from build123d import *

# Parameters (mm, degrees)
BOSS_EXTRUDE1_DEPTH     = 4
SKETCH1_4_R             = 4
BOSS_EXTRUDE2_DEPTH     = 27.15
FILLET3_SIZE            = 7.5
FILLET3_SIZE_2          = 10
CUT_EXTRUDE1_START      = -1.932
SKETCH6_R               = 4
SKETCH6_R_2             = 3.356
CUT_EXTRUDE1_DEPTH      = 1.932
SKETCH8_R               = 2.5
CUT_EXTRUDE3_DEPTH      = 5
CHAMFER1_SIZE           = 2
CHAMFER1_SIZE2          = 0.727940469
CUT_EXTRUDE2_DEPTH      = 36.735801376
CUT_EXTRUDE2_DEPTH_BACK = 36.735801376
SKETCH7_R               = 2.25
SKETCH13_W              = 0.25
SKETCH13_H              = 2.75
CHAMFER4_SIZE           = 0.3
CHAMFER4_SIZE_2         = 0.210062261
SKETCH10_W              = 3
SKETCH10_H              = 2
CUT_EXTRUDE15_DEPTH     = 1.5
CIRPATTERN2_COUNT       = 3
CUT_EXTRUDE16_START     = -1.932
SKETCH14_R              = 3.356
SKETCH14_R_2            = 2.3
CUT_EXTRUDE16_DEPTH     = 1.932


with BuildPart() as part:
    # Sketch1 → Boss-Extrude1 (new body)
    with BuildSketch(Plane(origin=(0, 0, 0), x_dir=(1, 0, 0), z_dir=(0, 1, 0))):
        with BuildLine():
            Line((-14.089714637, 3.515898385), (-18.307111179, 5.950813414))
            ThreePointArc((-18.307111179, 5.950813414), (-16.670989023, -9.625), (-4, -18.829830058))
            Line((-4, -18.829830058), (-4, -13.96))
            ThreePointArc((-4, -13.96), (-3.698779414, -12.437163552), (-2.840484577, -11.143681948))
            ThreePointArc((-2.840484577, -11.143681948), (0, -11.5), (2.840484577, -11.143681948))
            ThreePointArc((2.840484577, -11.143681948), (3.698779414, -12.437163552), (4, -13.96))
            Line((4, -13.96), (4, -18.829830058))
            ThreePointArc((4, -18.829830058), (16.670989023, -9.625), (18.307111179, 5.950813414))
            Line((18.307111179, 5.950813414), (14.089714637, 3.515898385))
            ThreePointArc((14.089714637, 3.515898385), (12.620289295, 3.015344841), (11.070953948, 3.111909171))
            ThreePointArc((11.070953948, 3.111909171), (9.959292144, 5.75), (8.230469371, 8.031772777))
            ThreePointArc((8.230469371, 8.031772777), (8.92150988, 9.421818712), (10.089714637, 10.444101615))
            Line((10.089714637, 10.444101615), (14.307111179, 12.879016644))
            ThreePointArc((14.307111179, 12.879016644), (0, 19.25), (-14.307111179, 12.879016644))
            Line((-14.307111179, 12.879016644), (-10.089714637, 10.444101615))
            ThreePointArc((-10.089714637, 10.444101615), (-8.92150988, 9.421818712), (-8.230469371, 8.031772777))
            ThreePointArc((-8.230469371, 8.031772777), (-9.959292144, 5.75), (-11.070953948, 3.111909171))
            ThreePointArc((-11.070953948, 3.111909171), (-12.620289295, 3.015344841), (-14.089714637, 3.515898385))
        make_face()
    extrude(amount=-BOSS_EXTRUDE1_DEPTH)

    # Sketch1<4> → Boss-Extrude2 (add)
    with BuildSketch(Plane(origin=(0, 0, 0), x_dir=(1, 0, 0), z_dir=(0, 1, 0))):
        with Locations(Location((0, 0, 0), (0, 0, 270))):
            Circle(SKETCH1_4_R)
    extrude(amount=-BOSS_EXTRUDE2_DEPTH)

    # Sketch2 → Cut-Revolve4 (revolve, cut)
    with BuildSketch(Plane(origin=(0, 0, 0), x_dir=(0, 0, -1), z_dir=(1, 0, 0)), mode=Mode.PRIVATE) as cut_revolve4_sk:
        Polygon((0, -27.15), (2.3, -27.15), (2.3, -25.15), (2.5, 0), (0, 0), align=None)
    revolve(cut_revolve4_sk.sketch.rotate(Axis((0, 0, 0), (0, -1, 0)), 180), axis=Axis((0, 0, 0), (0, -1, 0)), mode=Mode.SUBTRACT)

    # Fillet3
    # an asymmetric fillet: 10, 7.5 mm, written as the material it adds along each edge
    with BuildSketch(Plane(origin=(0, -4, 0), x_dir=(0, 0, 1), z_dir=(-1, 0, 0))) as fillet3_piece_1_section:
        with BuildLine():
            Bezier((4 + FILLET3_SIZE, 0), (4, 0), (4, -FILLET3_SIZE_2), weights=[1, 0.707106781, 1])
            Line((4, -FILLET3_SIZE_2), (4, 0))
            Line((4, 0), (4 + FILLET3_SIZE, 0))
        make_face()
    fillet3_piece_1 = revolve(axis=Axis((0, -4, 0), (0, 1, 0)), mode=Mode.PRIVATE)
    fillet3_piece_1 = fillet3_piece_1 & Plane(origin=(0, -3.929777006, 0), x_dir=(-0.7156929887401748, 0, -0.6984150240853615), z_dir=(0, 1, 0)) * Cylinder(11.5, 46, mode=Mode.PRIVATE)
    add(fillet3_piece_1)

    # Sketch5 → Cut-Revolve8 (revolve, cut)
    with BuildSketch(Plane.XY, mode=Mode.PRIVATE) as cut_revolve8_sk:
        Polygon((0, -7), (0, -9.309401077), (-4.55, -6.682457352), (-4.55, 0), (-2.55, 0), (-2.55, -5.527756814), align=None)
        Polygon((0, 0), (0, -7), (-2.55, -5.527756814), (-2.55, 0), align=None)
    revolve(cut_revolve8_sk.sketch.rotate(Axis((0, 0, 0), (0, -1, 0)), 270), axis=Axis((0, 0, 0), (0, -1, 0)), mode=Mode.SUBTRACT)

    # Sketch6 → Cut-Extrude1 (cut)
    with BuildSketch(Plane.XZ.offset(27.15).offset(CUT_EXTRUDE1_START)):
        with Locations(Location((0, 0, 0), (0, 0, 90))):
            Circle(SKETCH6_R)
        with Locations(Location((0, 0, 0), (0, 0, 270))):
            Circle(SKETCH6_R_2, mode=Mode.SUBTRACT)
    extrude(amount=CUT_EXTRUDE1_DEPTH, mode=Mode.SUBTRACT)

    # Sketch8 → Cut-Extrude3 (cut)
    with BuildSketch(Plane(origin=(0, -23, 0), x_dir=(1, 0, 0), z_dir=(0, 1, 0))):
        with Locations((0, 4)):
            Circle(SKETCH8_R)
    extrude(amount=CUT_EXTRUDE3_DEPTH, mode=Mode.SUBTRACT)

    # Chamfer1
    chamfer1_edges = [part.edges().sort_by_distance(p)[0] for p in [
        (0, -18, -4),
    ]]
    chamfer1_side = [part.faces().sort_by_distance(p)[0] for p in [
        (0, -19.609, -4),
    ]]
    chamfer(chamfer1_edges, length=CHAMFER1_SIZE, length2=CHAMFER1_SIZE2, reference=chamfer1_side[0])

    # Sketch7 → Cut-Extrude2 (cut, two sides: drawn at the far end of the back side and taken through both)
    with BuildSketch(Plane.XZ.offset(4).offset(-CUT_EXTRUDE2_DEPTH_BACK)):
        with Locations(Location((0, -6.25, 0), (0, 0, 56.387449327))):
            Circle(SKETCH7_R)
    extrude(amount=CUT_EXTRUDE2_DEPTH + CUT_EXTRUDE2_DEPTH_BACK, mode=Mode.SUBTRACT)

    # Sketch13 → Cut-Revolve14 (revolve, cut)
    with BuildSketch(Plane(origin=(0, 0, 0), x_dir=(0, 0, -1), z_dir=(1, 0, 0)), mode=Mode.PRIVATE) as cut_revolve14_sk:
        with Locations((-3.875, -20.5)):
            Rectangle(SKETCH13_W, SKETCH13_H)
    revolve(cut_revolve14_sk.sketch.rotate(Axis((0, -7.902306907, 0), (0, -1, 0)), 216.419913729), axis=Axis((0, -7.902306907, 0), (0, -1, 0)), mode=Mode.SUBTRACT)

    # Chamfer4
    # the kernel refuses this chamfer: 0.3, 0.210062261 mm, written as the material it adds along each edge
    with BuildSketch(Plane(origin=(0, -21.875, 0), x_dir=(0.43172798800380885, 0, -0.9020038494231514), z_dir=(-0.9020038494231514, 0, -0.43172798800380885))) as chamfer4_piece_1_section:
        Polygon((3.75 + CHAMFER4_SIZE, 0), (3.75, -CHAMFER4_SIZE_2 * 1.0000000022), (3.75, 0), align=None)
    chamfer4_piece_1 = revolve(axis=Axis((0, -21.875, 0), (0, -1, 0)), revolution_arc=308.845454641, mode=Mode.PRIVATE)
    chamfer4_piece_1 = chamfer4_piece_1 & Plane(origin=(0, -21.756112084, 0), x_dir=(0, 0, 1), z_dir=(0, 1, 0)) * Cylinder(4, 17, mode=Mode.PRIVATE)
    chamfer4_piece_1 = chamfer4_piece_1 - Plane(origin=(0, -21.756112084, -4), x_dir=(1, 0, 0), z_dir=(0, -1, 0)) * Cylinder(2.5, 17, mode=Mode.PRIVATE)
    add(chamfer4_piece_1)

    # Sketch10 → Cut-Extrude15 (cut, symmetric)
    with BuildSketch(Plane(origin=(0, 0, 0), x_dir=(0, 0, -1), z_dir=(1, 0, 0))):
        with Locations((-11.46, -2)):
            Rectangle(SKETCH10_W, SKETCH10_H)
        Polygon((-4.55, -4), (-9.96, -3), (-9.96, -1), (-4.55, -2), align=None)
        with Locations((-3.05, -3)):
            Rectangle(SKETCH10_W, SKETCH10_H)
    cut_extrude15 = extrude(amount=CUT_EXTRUDE15_DEPTH, both=True, mode=Mode.SUBTRACT)

    # CirPattern2: Cut-Extrude15 ×3 about axis
    cirpattern2_axis = Axis((0, 0, 0), (0, 1, 0))
    for i in range(1, CIRPATTERN2_COUNT):
        add(cut_extrude15.rotate(cirpattern2_axis, i * 360 / CIRPATTERN2_COUNT), mode=Mode.SUBTRACT)

    # Sketch14 → Cut-Extrude16 (cut)
    with BuildSketch(Plane.XZ.offset(27.15).offset(CUT_EXTRUDE16_START)):
        Circle(SKETCH14_R)
        with Locations(Location((0, 0, 0), (0, 0, 90))):
            Circle(SKETCH14_R_2, mode=Mode.SUBTRACT)
    extrude(amount=CUT_EXTRUDE16_DEPTH, mode=Mode.SUBTRACT)


solid = part.part
Work out the finished part from the listing and answer in its coordinate system (mm). A direction names the side the tool comes from. Coordinates: 2 decimals unless noted, no trailing zeros. Write each loop counter-clockwise with the first axis right and the second up, starting at its lowest first coordinate (ties: lowest second). Pieces come first, ordered by that corner, then holes. Notation, with made-up numbers: M -19,-11 L 30,-11 A28 ccw 30,21 Z; hole C 18.5,27.5 d9. An arc over 180 degrees is marked long. Write item = value, one per line.
1. For faces 1 (the face through (-1.532, -16.527, 3.695)), 2 (the face through (6.305, -1.493, -3.665)), 3 (the face through (0, -1, 11)), 4 (the face through (-12.599, -1.972, -3.013)), determine the directions among +Z, -Z, +X, -X, +Y, -Y from which every point of the face is accessible in a straight line to the end or side of a thin tool.
Solution:
face_1 = -Y
face_2 = none
face_3 = +Z
face_4 = +Y, -Y
2. The part is cut by section A-A (x = -12). Determine the outline of the cut face in (y, z).
Solution:
outline = M -4,-15.05 L 0,-15.05 L 0,-11.55 L -4,-11.55 Z; M -4,-2.98 L 0,-2.98 L 0,15.05 L -4,15.05 Z
3. The part is cut by section C-C (z = -16). Determine the outline of the cut face in (x, y).
Solution:
outline = M -10.7,-4 L 10.7,-4 L 10.7,0 L -10.7,0 Z
4. The part is cut by section D-D (x = 17). Determine the outline of the cut face in (y, z).
Solution:
outline = M -4,-5.2 L 0,-5.2 L 0,9.03 L -4,9.03 Z
5. Determine the mould class of faces 5 (the face through (12.169, -1.972, -11.645)), 6 (the face through (0, -4, -14)), 7 (the face through (0.131, -20.377, 3.748)) for opening direction Y: released by +Y, released by -Y, zero draft, split by the parting line, or undercut.
Solution:
face_5 = zero draft
face_6 = released by -Y
face_7 = undercut
6. The part is cut by section B-B (z = 15). Determine the outline of the cut face in (x, y), then the cut area to 3 significant figures.
Solution:
outline = M -12.06,-4 L -4,-4 L -4,0 L -12.06,0 Z; M 4,-4 L 12.06,-4 L 12.06,0 L 4,0 Z
area = 64.5 mm2
7. Straight lines are drawn through the part: line 1 (X direction, y = -25.15, z = 0); line 2 (X direction, y = -5, z = 0); line 3 (Y direction, x = -14.5, z = 11). For each, find the intervals that lie inside material, in ascending order. Write a range as from..to.
Solution:
line_1 = -4..-2.3, 2.3..4
line_2 = -8.23..-4.55, 4.55..8.23
line_3 = -4..0
8. Flat-ended cylindrical pins translate along their axes: pin 1 (1.2 mm diameter, centred on y = -2, z = 17, fed in from +X); pin 2 (0.8 mm diameter, centred on x = -9, z = -5.5, fed in from -Y); pin 3 (8 mm diameter, centred on x = 3, z = -5.5, fed in from -Y); pin 4 (6 mm diameter, centred on y = -9.5, z = 0.5, fed in from -X). Find the tip coordinate at first contact, or state that the pin passes through.
Solution:
pin_1 = 10.08
pin_2 = -4.16
pin_3 = -25.22
pin_4 = -6.53
